```python
from build123d import *

# Parameters (mm, degrees)
ESQUISSE1_R             = 22.5
ESQUISSE1_R_2           = 9.5
BOSS_EXTRU_1_DEPTH      = 40
BOSS_EXTRU_2_DEPTH      = 6.35
BOSS_EXTRU_2_DEPTH_BACK = 46.35
ESQUISSE2_R             = 9.5
ESQUISSE3_R             = 8
ENL_V_MAT_EXTRU_1_DEPTH = 194.400037211
ESQUISSE4_R             = 8
ENL_V_MAT_EXTRU_2_DEPTH = 184.407892092
ENL_V_START             = -9.5
ENL_V_MAT_EXTRU_3_DEPTH = 9.5


with BuildPart() as part:
    # Esquisse1 → Boss.-Extru.1 (new body)
    # profile 1 of 2: a face of its own
    with BuildSketch(Plane.XY):
        with BuildLine():
            ThreePointArc((0, -22.5), (-19.23551709, 11.672398309), (19.957743747, 10.389343798))
            Line((19.957743747, 10.389343798), (-17.289116996, 81.93989757))
            Line((-17.289116996, 81.93989757), (-28.376752411, 76.168039905))
            Line((-28.376752411, 76.168039905), (-50.695462776, 119.041883612))
            Line((-50.695462776, 119.041883612), (-68.435679439, 109.806911348))
            Line((-68.435679439, 109.806911348), (-46.116969074, 66.93306764))
            Line((-46.116969074, 66.93306764), (-88.25, 45))
            Line((-88.25, 45), (-88.25, 10))
            Line((-88.25, 10), (-140, 10))
            Line((-140, 10), (-140, -10))
            Line((-140, -10), (-88.25, -10))
            Line((-88.25, -10), (-88.25, -22.5))
            Line((-88.25, -22.5), (0, -22.5))
        make_face()
    # profile 2 of 2: a face of its own
    with BuildSketch(Plane.XY):
        Circle(ESQUISSE1_R)
        Circle(ESQUISSE1_R_2, mode=Mode.SUBTRACT)
    extrude(amount=BOSS_EXTRU_1_DEPTH)

    # Esquisse2 → Boss.-Extru.2 (add, two sides: drawn at the far end of the back side and taken through both)
    with BuildSketch(Plane.XY.offset(40).offset(-BOSS_EXTRU_2_DEPTH_BACK)):
        with BuildLine():
            ThreePointArc((19.957743747, 10.389343798), (-19.23551709, 11.672398309), (0, -22.5))
            ThreePointArc((0, -22.5), (15.909902577, -15.909902577), (22.5, 0))
            ThreePointArc((22.5, 0), (21.855196571, 5.347932577), (19.957743747, 10.389343798))
        make_face()
        Circle(ESQUISSE2_R, mode=Mode.SUBTRACT)
    extrude(amount=BOSS_EXTRU_2_DEPTH + BOSS_EXTRU_2_DEPTH_BACK)

    # Esquisse3 → Enlèv. mat.-Extru.1 (cut, through all)
    with BuildSketch(Plane(origin=(8.870108332, 4.617486132, 0), x_dir=(0, 0, -1), z_dir=(0.8870108331782226, 0.4617486132350323, 0))):
        with BuildLine():
            ThreePointArc((-20, 129), (-5.857864376, 123.142135624), (0, 109))
            Line((0, 109), (0, 129))
            Line((0, 129), (-20, 129))
        make_face()
        with BuildLine():
            ThreePointArc((-40, 109), (-34.142135624, 123.142135624), (-20, 129))
            Line((-20, 129), (-40, 129))
            Line((-40, 129), (-40, 109))
        make_face()
        with Locations(Location((-20, 109, 0), (0, 0, 90))):
            Circle(ESQUISSE3_R)
    extrude(amount=-ENL_V_MAT_EXTRU_1_DEPTH, mode=Mode.SUBTRACT)

    # Esquisse4 → Enlèv. mat.-Extru.2 (cut, through all)
    with BuildSketch(Plane(origin=(0, 10, 0), x_dir=(1, 0, 0), z_dir=(0, 1, 0))):
        with Locations(Location((-120, -20, 0), (0, 0, 180))):
            Circle(ESQUISSE4_R)
        with BuildLine():
            ThreePointArc((-140, -20), (-134.142135624, -5.857864376), (-120, 0))
            Line((-120, 0), (-140, 0))
            Line((-140, 0), (-140, -20))
        make_face()
        with BuildLine():
            ThreePointArc((-120, -40), (-134.142135624, -34.142135624), (-140, -20))
            Line((-140, -20), (-140, -40))
            Line((-140, -40), (-120, -40))
        make_face()
    extrude(amount=-ENL_V_MAT_EXTRU_2_DEPTH, mode=Mode.SUBTRACT)

    # Esquisse5 → Enlèv. mat.-Extru.3 (cut)
    with BuildSketch(Plane.XY.offset(40).offset(ENL_V_START)):
        with BuildLine():
            ThreePointArc((-18.275239397, -13.125), (-20.943719878, -10.826826092), (-24.366985862, -10))
            Line((-24.366985862, -10), (-71.25, -10))
            ThreePointArc((-71.25, -10), (-76.553300859, -12.196699141), (-78.75, -17.5))
            Line((-78.75, -17.5), (-78.75, -22.5))
            Line((-78.75, -22.5), (0, -22.5))
            ThreePointArc((0, -22.5), (-10.269797953, -20.019521723), (-18.275239397, -13.125))
        make_face()
        with BuildLine():
            ThreePointArc((-2.381313599, 26.231266564), (-0.067221577, 23.576578352), (3.203450738, 22.270785872))
            ThreePointArc((3.203450738, 22.270785872), (13.01546768, 18.353408432), (19.957743747, 10.389343798))
            Line((19.957743747, 10.389343798), (-12.90250517, 73.513294655))
            Line((-12.90250517, 73.513294655), (-17.337559336, 71.204551589))
            ThreePointArc((-17.337559336, 71.204551589), (-21.027321868, 66.807263836), (-20.527025986, 61.08885574))
            Line((-20.527025986, 61.08885574), (-2.381313599, 26.231266564))
        make_face()
        with BuildLine():
            Line((-78.75, 17.5), (-78.75, 34.684146763))
            ThreePointArc((-78.75, 34.684146763), (-77.66183903, 38.574946199), (-74.713114599, 41.336728011))
            Line((-74.713114599, 41.336728011), (-48.382938497, 55.043350125))
            ThreePointArc((-48.382938497, 55.043350125), (-42.664530402, 55.543646007), (-38.267242649, 51.853883476))
            Line((-38.267242649, 51.853883476), (-22.186526206, 20.963114599))
            ThreePointArc((-22.186526206, 20.963114599), (-22.427268425, 13.609200564), (-28.839107455, 10))
            Line((-28.839107455, 10), (-71.25, 10))
            ThreePointArc((-71.25, 10), (-76.553300859, 12.196699141), (-78.75, 17.5))
        make_face()
    enl_v_mat_extru_3 = extrude(amount=ENL_V_MAT_EXTRU_3_DEPTH, mode=Mode.SUBTRACT)

    # Symétrie1: Enlèv. mat.-Extru.3 across plane
    add(enl_v_mat_extru_3.mirror(Plane(origin=(0, 0, 20), x_dir=(1, 0, 0), z_dir=(0, 0, -1))), mode=Mode.SUBTRACT)


solid = part.part
```
Here's how the part is built. I have some questions about the finished solid (model axes, mm). A direction names the side the tool comes from. Round coordinates to 2 decimals unless told otherwise and drop trailing zeros. One line per question, with ' | ' between items.
1) If we mould it in two halves opening along X, with no side actions, what happens to faces 1 (the face through (-78.75, -20, 35)), 2 (the face through (-88.25, 28, 20)), 3 (the face through (-20.9, -10.85, 35.18)), 4 (the face through (-59, 8, 0))? For each: +X half, -X half, draft (parallel to the pull), parting line (faces both ways), or undercut.
Working result:
face 1: undercut | face 2: -X half | face 3: undercut | face 4: draft
2) For pin 1 Ø6 at (x, z) = (-117.5, 27) entering from -Y; pin 2 Ø14 at (y, z) = (-16.5, 17) entering from -X; pin 3 Ø10 at (x, y) = (-24, -14.5) entering from -Z, each with a flat end and sliding along its axis, tell me the tip position at first contact or that it passes through.
Working result:
pin 1: y = -10 | pin 2: x = -140 | pin 3: z = 0
3) I want a section at A-A, the plane z = 36.5. State how many separate pieces and enclosed holes the cut face has, then the cut area to 3 significant figures.
Working result:
separate pieces: 1 | enclosed holes: 2 | area: 6,520 mm²
4) I need wall thicknesses on line 1 along Z through (x, y) = (-120, 1.75); line 2 along Y through (x, z) = (-116, 31); line 3 along Z through (x, y) = (-25.5, 13.5). Which ranges of each line are inside material? Lowest first, please.
Working result:
line 1: 0 to 12, 28 to 40 | line 2: -10 to 10 | line 3: 9.5 to 30.5
5) For faces 5 (the face through (-36.9, 92.54, 19.72)), 6 (the face through (-78.75, -20, 5)), 7 (the face through (-22.372, 13.702, 35.184)), which set-ups out of +Z, -Z, +X, -X, +Y, -Y let a thin tool reach every point of the face, with its end or its side?
Working result:
face 5: +Z, -Z, +Y | face 6: -Z, -Y | face 7: +Z
